Model file for the job. Use its own axes, mm. Round coordinates to 2 decimals unless told otherwise and drop trailing zeros. Order: outer loops, then holes, each group sorted by start corner. A loop starts at its lowest first (then second) coordinate and runs counter-clockwise, first axis right, second up. Notation, with made-up numbers: (75.5, 63.25) - (90.5, 63.25) arc R17 cw to (90.5, 68.25) - close; hole circle Ø2 at (61, 75.25). An arc over 180 degrees is marked (long way). Put each result on its own line as item: value. Start each with the question number.
Item 1: Pin check, flat tips, straight feed: pin 1 Ø1 at (y, z) = (2, 1.5) entering from +X; pin 2 Ø1.6 at (x, y) = (-59, 1.5) entering from +Z; pin 3 Ø1 at (x, y) = (58, 2) entering from -Z. Stop position of each tip, or through.
Item 2: Saw through at B-B on z = 5. List the corners of the cut face in (x, y) (3 decimals), plus the area to 3 significant figures.
Item 3: Saw through at C-C on y = 1.05. State how many separate pieces and enclosed holes the cut face has, plus the area to 3 significant figures.
Item 4: Probe probe 1 along X at (y, z) = (0.9, -2); probe 2 along Z at (x, y) = (0, 1.15); probe 3 along Z at (x, y) = (-22, 2.95). List the from-to ranges inside material, lowest first.
Item 5: Saw through at A-A on x = 0. List the corners of the cut face in (y, z) (3 decimals).
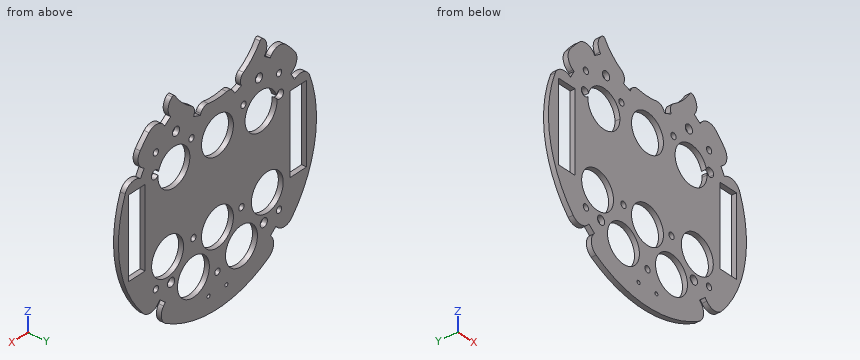
```python
from build123d import *

# Parameters (mm, degrees)
SKETCH1_R           = 2
SKETCH1_R_2         = 2.75
SKETCH1_W           = 12.7
SKETCH1_H           = 50.8
SKETCH1_R_3         = 12.095
SKETCH1_R_4         = 12.075
SKETCH1_R_5         = 1.143
BOSS_EXTRUDE1_DEPTH = 3.175


with BuildPart() as part:
    # Sketch1 → Boss-Extrude1 (new body)
    with BuildSketch(Plane(origin=(0, 0, 0), x_dir=(1, 0, 0), z_dir=(0, 1, 0))):
        with BuildLine():
            Line((-35.441180971, -55.409730648), (-36.014757408, -56.228882693))
            ThreePointArc((-36.014757408, -56.228882693), (-37.282182463, -61.682274385), (-34.419720881, -66.493943628))
            ThreePointArc((-34.419720881, -66.493943628), (-33.243515234, -66.777434912), (-32.240681933, -66.10056535))
            ThreePointArc((-32.240681933, -66.10056535), (-26.728650164, -59.250774979), (-19.793246149, -53.846860332))
            ThreePointArc((-19.793246149, -53.846860332), (-17.659799789, -51.192486841), (-17.721018114, -47.787557426))
            Line((-17.721018114, -47.787557426), (-18.078412971, -46.853604046))
            Line((-18.078412971, -46.853604046), (-12.941669381, -44.887932332))
            Line((-12.941669381, -44.887932332), (-12.584274523, -45.821885712))
            ThreePointArc((-12.584274523, -45.821885712), (-10.356790186, -48.397852623), (-6.996351286, -48.949887413))
            ThreePointArc((-6.996351286, -48.949887413), (0, -48.302004425), (6.996351286, -48.949887413))
            ThreePointArc((6.996351286, -48.949887413), (10.356790186, -48.397852623), (12.584274523, -45.821885712))
            Line((12.584274523, -45.821885712), (12.941669381, -44.887932332))
            Line((12.941669381, -44.887932332), (18.078412971, -46.853604046))
            Line((18.078412971, -46.853604046), (17.721018114, -47.787557426))
            ThreePointArc((17.721018114, -47.787557426), (17.659799789, -51.192486841), (19.793246149, -53.846860332))
            ThreePointArc((19.793246149, -53.846860332), (26.728650164, -59.250774979), (32.240681933, -66.10056535))
            ThreePointArc((32.240681933, -66.10056535), (33.243515234, -66.777434912), (34.419720881, -66.493943628))
            ThreePointArc((34.419720881, -66.493943628), (37.282182463, -61.682274385), (36.014757408, -56.228882693))
            Line((36.014757408, -56.228882693), (35.441180971, -55.409730648))
            Line((35.441180971, -55.409730648), (39.946517215, -52.255060248))
            Line((39.946517215, -52.255060248), (40.520093651, -53.074212293))
            ThreePointArc((40.520093651, -53.074212293), (45.927580176, -56.23617342), (51.848593315, -54.191543356))
            ThreePointArc((51.848593315, -54.191543356), (55.295899374, -50.669157408), (58.504414423, -46.927960674))
            ThreePointArc((58.504414423, -46.927960674), (60.025192689, -40.851285995), (56.403972981, -35.739974078))
            Line((56.403972981, -35.739974078), (55.537947577, -35.239974078))
            Line((55.537947577, -35.239974078), (58.287686569, -30.477286437))
            Line((58.287686569, -30.477286437), (59.153711973, -30.977286437))
            ThreePointArc((59.153711973, -30.977286437), (65.390847794, -31.557698738), (69.893013303, -27.202328787))
            ThreePointArc((69.893013303, -27.202328787), (73.860606951, 13.023468848), (56.374397975, 49.466425512))
            ThreePointArc((56.374397975, 49.466425512), (50.654117331, 52.01932544), (44.991624855, 49.340690033))
            Line((44.991624855, 49.340690033), (43.706049635, 47.808601147))
            Line((43.706049635, 47.808601147), (39.492805198, 51.343933))
            Line((39.492805198, 51.343933), (40.778380417, 52.876021886))
            ThreePointArc((40.778380417, 52.876021886), (42.433039833, 58.917628536), (38.925607882, 64.107698843))
            ThreePointArc((38.925607882, 64.107698843), (0, 75), (-38.925607882, 64.107698843))
            ThreePointArc((-38.925607882, 64.107698843), (-42.433039833, 58.917628536), (-40.778380417, 52.876021886))
            Line((-40.778380417, 52.876021886), (-40.135592808, 52.109977443))
            Line((-40.135592808, 52.109977443), (-44.348837245, 48.57464559))
            Line((-44.348837245, 48.57464559), (-44.991624855, 49.340690033))
            ThreePointArc((-44.991624855, 49.340690033), (-50.654117331, 52.01932544), (-56.374397975, 49.466425512))
            ThreePointArc((-56.374397975, 49.466425512), (-73.860606951, 13.023468848), (-69.893013303, -27.202328787))
            ThreePointArc((-69.893013303, -27.202328787), (-65.390847794, -31.557698738), (-59.153711973, -30.977286437))
            Line((-59.153711973, -30.977286437), (-58.287686569, -30.477286437))
            Line((-58.287686569, -30.477286437), (-55.537947577, -35.239974078))
            Line((-55.537947577, -35.239974078), (-56.403972981, -35.739974078))
            ThreePointArc((-56.403972981, -35.739974078), (-60.025192689, -40.851285995), (-58.504414423, -46.927960674))
            ThreePointArc((-58.504414423, -46.927960674), (-55.295899374, -50.669157408), (-51.848593315, -54.191543356))
            ThreePointArc((-51.848593315, -54.191543356), (-45.927580176, -56.23617342), (-40.520093651, -53.074212293))
            Line((-40.520093651, -53.074212293), (-39.946517215, -52.255060249))
            Line((-39.946517215, -52.255060249), (-35.441180971, -55.409730648))
        make_face()
        with Locations((-46.663733983, -40.081231883)):
            Circle(SKETCH1_R, mode=Mode.SUBTRACT)
        with Locations((-31.384508293, -44.821722961)):
            Circle(SKETCH1_R_2, mode=Mode.SUBTRACT)
        with Locations((-19.709430746, -34.896815973)):
            Circle(SKETCH1_R, mode=Mode.SUBTRACT)
        with Locations((-61.164123727, 0)):
            Rectangle(SKETCH1_W, SKETCH1_H, mode=Mode.SUBTRACT)
        with BuildLine():
            ThreePointArc((-45.027393846, -25.827452847), (-33.613665776, -12.513676165), (-20.900567885, -24.59287233))
            ThreePointArc((-20.900567885, -24.59287233), (-31.339636328, -36.573978943), (-44.637139307, -27.873549061))
            ThreePointArc((-44.637139307, -27.873549061), (-50.033654419, -27.842568285), (-45.027393846, -25.827452847))
        make_face(mode=Mode.SUBTRACT)
        with Locations((31.384508293, -44.821722961)):
            Circle(SKETCH1_R_2, mode=Mode.SUBTRACT)
        with Locations((19.709430746, -34.896815973)):
            Circle(SKETCH1_R, mode=Mode.SUBTRACT)
        with Locations((46.663733983, -40.081231883)):
            Circle(SKETCH1_R, mode=Mode.SUBTRACT)
        with Locations((0, -26.93833729)):
            Circle(SKETCH1_R_3, mode=Mode.SUBTRACT)
        with BuildLine():
            ThreePointArc((44.637139307, -27.873549061), (21.014461272, -22.936940773), (45.090567885, -24.59287233))
            ThreePointArc((45.090567885, -24.59287233), (45.07476405, -25.210970221), (45.027393846, -25.827452847))
            ThreePointArc((45.027393846, -25.827452847), (48.114612939, -24.690952678), (50.082350097, -27.32734507))
            ThreePointArc((50.082350097, -27.32734507), (47.606822617, -30.063613484), (44.637139307, -27.873549061))
        make_face(mode=Mode.SUBTRACT)
        with Locations((61.164123727, 0)):
            Rectangle(SKETCH1_W, SKETCH1_H, mode=Mode.SUBTRACT)
        with Locations((-37.772386795, 25.4)):
            Circle(SKETCH1_R_4, mode=Mode.SUBTRACT)
        with Locations((-18.178952795, 24.310551096)):
            Circle(SKETCH1_R, mode=Mode.SUBTRACT)
        with Locations((-46.663733983, 40.081231883)):
            Circle(SKETCH1_R, mode=Mode.SUBTRACT)
        with Locations((-35.134053633, 41.871134639)):
            Circle(SKETCH1_R_2, mode=Mode.SUBTRACT)
        with Locations((-18.1962694, 47.04580506)):
            Circle(SKETCH1_R_3, mode=Mode.SUBTRACT)
        with Locations((-6.731, 64.107698843)):
            Circle(SKETCH1_R_5, mode=Mode.SUBTRACT)
        with Locations((0, 26.93833729)):
            Circle(SKETCH1_R_3, mode=Mode.SUBTRACT)
        with Locations((18.178952795, 24.310551096)):
            Circle(SKETCH1_R, mode=Mode.SUBTRACT)
        with Locations((37.772386795, 25.4)):
            Circle(SKETCH1_R_3, mode=Mode.SUBTRACT)
        with Locations((18.1962694, 47.04580506)):
            Circle(SKETCH1_R_3, mode=Mode.SUBTRACT)
        with Locations((0, 53.061187965)):
            Circle(SKETCH1_R, mode=Mode.SUBTRACT)
        with Locations((35.134053633, 41.871134639)):
            Circle(SKETCH1_R_2, mode=Mode.SUBTRACT)
        with Locations((6.731, 64.107698843)):
            Circle(SKETCH1_R_5, mode=Mode.SUBTRACT)
        with Locations((46.663733983, 40.081231883)):
            Circle(SKETCH1_R, mode=Mode.SUBTRACT)
    extrude(amount=BOSS_EXTRUDE1_DEPTH)


solid = part.part
```
Results found:
1. pin 1: stops at x = 74.99
1. pin 2: stops at z = 47.3
1. pin 3: stops at z = -48.15
2. outline: (-74.833, 0) - (-67.514, 0) - (-67.514, 3.175) - (-74.833, 3.175) - close; (-54.814, 0) - (54.814, 0) - (54.814, 3.175) - (-54.814, 3.175) - close; (67.514, 0) - (74.833, 0) - (74.833, 3.175) - (67.514, 3.175) - close
2. area: 395 mm²
3. separate pieces: 1
3. enclosed holes: 25
3. area: 10,600 mm²
4. probe 1: x = -74.97 to -67.51, -54.81 to 54.81, 67.51 to 74.97
4. probe 2: z = -75 to -55.06, -51.06 to -39.03, -14.84 to 14.84, 39.03 to 48.3
4. probe 3: z = -71.7 to -58.53, -35.56 to 19.55, 29.63 to 55.3
5. outline: (0, -75) - (3.175, -75) - (3.175, -55.061) - (0, -55.061) - close; (0, -51.061) - (3.175, -51.061) - (3.175, -39.033) - (0, -39.033) - close; (0, -14.843) - (3.175, -14.843) - (3.175, 14.843) - (0, 14.843) - close; (0, 39.033) - (3.175, 39.033) - (3.175, 48.302) - (0, 48.302) - close
